```python
from build123d import *

# Parameters (mm, degrees)
SKETCH1_W           = 155
SKETCH1_H           = 55
BOSS_EXTRUDE1_DEPTH = 10
SKETCH2_W           = 143
SKETCH2_H           = 20
CUT_EXTRUDE1_DEPTH  = 5
SKETCH3_W           = 10
SKETCH3_H           = 30
BOSS_EXTRUDE2_DEPTH = 78
SKETCH4_W           = 35
SKETCH4_H           = 20
SKETCH4_W_2         = 50
CUT_EXTRUDE2_DEPTH  = 78
SKETCH5_W           = 155
SKETCH5_H           = 88
BOSS_EXTRUDE3_DEPTH = 15
SKETCH6_W           = 115
SKETCH6_H           = 48
CUT_EXTRUDE3_DEPTH  = 20
SKETCH7_W           = 5
SKETCH7_H           = 58
CUT_EXTRUDE4_DEPTH  = 200
CUT_EXTRUDE5_DEPTH  = 35
SKETCH9_R           = 2
CUT_EXTRUDE6_DEPTH  = 10
SKETCH10_R          = 2
CUT_EXTRUDE7_DEPTH  = 20


with BuildPart() as part:
    # Sketch1 → Boss-Extrude1 (new body)
    with BuildSketch(Plane(origin=(0, 0, 0), x_dir=(1, 0, 0), z_dir=(0, 1, 0))):
        with Locations((77.5, -27.5)):
            Rectangle(SKETCH1_W, SKETCH1_H)
    extrude(amount=BOSS_EXTRUDE1_DEPTH)

    # Sketch2 → Cut-Extrude1 (cut)
    with BuildSketch(Plane(origin=(0, 10, 0), x_dir=(1, 0, 0), z_dir=(0, 1, 0))):
        with Locations((77.5, -15)):
            Rectangle(SKETCH2_W, SKETCH2_H)
    extrude(amount=-CUT_EXTRUDE1_DEPTH, mode=Mode.SUBTRACT)

    # Sketch3 → Boss-Extrude2 (add)
    with BuildSketch(Plane(origin=(0, 10, 0), x_dir=(1, 0, 0), z_dir=(0, 1, 0))):
        with Locations((5, -40)):
            Rectangle(SKETCH3_W, SKETCH3_H)
        with Locations((150, -40)):
            Rectangle(SKETCH3_W, SKETCH3_H)
    extrude(amount=BOSS_EXTRUDE2_DEPTH)

    # Sketch4 → Cut-Extrude2 (cut)
    with BuildSketch(Plane(origin=(0, 5, 0), x_dir=(1, 0, 0), z_dir=(0, 1, 0))):
        with Locations((23.5, -15)):
            Rectangle(SKETCH4_W, SKETCH4_H)
        with Locations((124, -15)):
            Rectangle(SKETCH4_W_2, SKETCH4_H)
    extrude(amount=-CUT_EXTRUDE2_DEPTH, mode=Mode.SUBTRACT)

    # Sketch5 → Boss-Extrude3 (add)
    with BuildSketch(Plane.XY.offset(55)):
        with Locations((77.5, 44)):
            Rectangle(SKETCH5_W, SKETCH5_H)
    extrude(amount=BOSS_EXTRUDE3_DEPTH)

    # Sketch6 → Cut-Extrude3 (cut)
    with BuildSketch(Plane.XY.offset(70)):
        with Locations((77.5, 44)):
            Rectangle(SKETCH6_W, SKETCH6_H)
    extrude(amount=-CUT_EXTRUDE3_DEPTH, mode=Mode.SUBTRACT)

    # Sketch7 → Cut-Extrude4 (cut)
    with BuildSketch(Plane(origin=(155, 0, 0), x_dir=(0, 0, -1), z_dir=(1, 0, 0))):
        with Locations((-62.5, 44)):
            Rectangle(SKETCH7_W, SKETCH7_H)
    extrude(amount=-CUT_EXTRUDE4_DEPTH, mode=Mode.SUBTRACT)

    # Sketch8 → Cut-Extrude5 (cut)
    with BuildSketch(Plane.XY.offset(70)):
        Polygon((47.5, 0), (107.5, 0), (77.5, 50), align=None)
    extrude(amount=-CUT_EXTRUDE5_DEPTH, mode=Mode.SUBTRACT)

    # Sketch9 → Cut-Extrude6 (cut)
    with BuildSketch(Plane(origin=(0, 88, 0), x_dir=(1, 0, 0), z_dir=(0, 1, 0))):
        with Locations((150, -40)):
            Circle(SKETCH9_R)
        with Locations((5, -40)):
            Circle(SKETCH9_R)
    extrude(amount=-CUT_EXTRUDE6_DEPTH, mode=Mode.SUBTRACT)

    # Sketch10 → Cut-Extrude7 (cut)
    with BuildSketch(Plane(origin=(0, 88, 0), x_dir=(1, 0, 0), z_dir=(0, 1, 0))):
        with Locations((109, -62.5)):
            Circle(SKETCH10_R)
        with Locations((46, -62.5)):
            Circle(SKETCH10_R)
    extrude(amount=-CUT_EXTRUDE7_DEPTH, mode=Mode.SUBTRACT)


solid = part.part
```
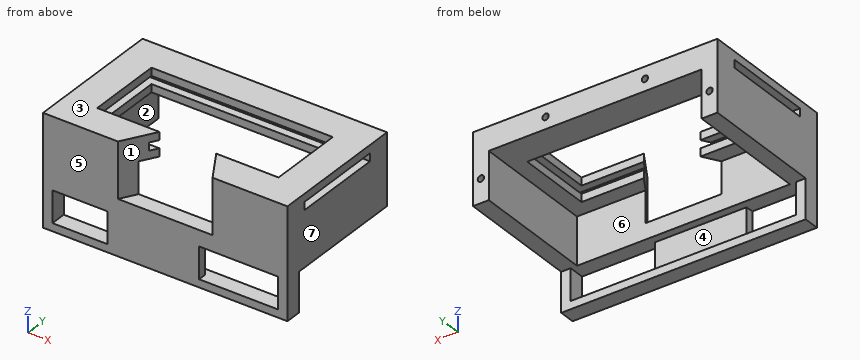
Can you work these out from the model? Positions are in its coordinate system, mm. Face numbers are marked on the shaded views. A direction names the side the tool comes from. Coordinates: 2 decimals unless noted, no trailing zeros. Write each loop counter-clockwise with the first axis right and the second up, starting at its lowest first coordinate (ties: lowest second). Pieces come first, ordered by that corner, then holes. Notation, with made-up numbers: (10.5, 78.25) - (50.5, 78.25) arc R30 ccw to (50.5, 107.25) - close; hole circle Ø11 at (36, 24). An arc over 180 degrees is marked (long way). Return JSON: item names as keys, results as strings.
Q1. I'm going to push flat-ended pins straight in: pin 1 Ø6 at (x, z) = (96.5, 17.5) entering from +Y; pin 2 Ø2 at (x, z) = (5.5, 40) entering from +Y; pin 3 Ø1.5 at (x, z) = (71, 68.5) entering from -Y; pin 4 Ø3 at (x, y) = (96, 65) entering from -Z. Where does each tip first touch, or does it pass through?
Computed values:
{"pin 1": "stops at y = 5", "pin 2": "stops at y = 78", "pin 3": "stops at y = 68", "pin 4": "passes through"}
Q2. If we section it at B-B (y = 59.5): Please give me the cut outline in (x, z), then the cut area to 3 significant figures.
Computed values:
{"outline": "(0, 25) - (10, 25) - (10, 55) - (20, 55) - (20, 60) - (0, 60) - close; (0, 65) - (20, 65) - (20, 70) - (0, 70) - close; (135, 55) - (145, 55) - (145, 25) - (155, 25) - (155, 60) - (135, 60) - close; (135, 65) - (155, 65) - (155, 70) - (135, 70) - close", "area": "1,000 mm2"}
Q3. If we section it at D-D (z = 9): Please give me the cut outline in (x, y).
Computed values:
{"outline": "(0, 0) - (6, 0) - (6, 10) - (0, 10) - close; (41, 0) - (99, 0) - (99, 5) - (41, 5) - close; (149, 0) - (155, 0) - (155, 10) - (149, 10) - close"}
Q4. Thinking about a two-plate mould opening in X: for the marked faces 5, 6 and 7, which applies, +X half, -X half, draft (parallel to the pull), parting line (faces both ways), or undercut?
Computed values:
{"face 5": "draft", "face 6": "undercut", "face 7": "+X half"}
Q5. If we section it at A-A (x = 76.5): Please give me the cut outline in (y, z).
Computed values:
{"outline": "(0, 0) - (10, 0) - (10, 5) - (5, 5) - (5, 25) - (10, 25) - (10, 35) - (0, 35) - close; (68, 55) - (88, 55) - (88, 70) - (68, 70) - (68, 65) - (73, 65) - (73, 60) - (68, 60) - close"}
Q6. If we section it at C-C (z = 40): Please give me the cut outline in (x, y).
Computed values:
{"outline": "(0, 0) - (47.5, 0) - (53.5, 10) - (10, 10) - (10, 88) - (7, 88) - (7, 78) - (3, 78) - (3, 88) - (0, 88) - close; (101.5, 10) - (107.5, 0) - (155, 0) - (155, 88) - (152, 88) - (152, 78) - (148, 78) - (148, 88) - (145, 88) - (145, 10) - close"}
Q7. Please list where these lines run through material, in increasing order: L1, parallel to X at y = 84.75, z = 40; L2, parallel to X at y = 69, z = 37; L3, parallel to Z at x = 109, y = 84.5. Write a range as from..to.
Computed values:
{"L1": "x = 0..3, 7..10, 145..148, 152..155", "L2": "x = 0..10, 145..155", "L3": "z = 55..60.5, 64.5..70"}
Q8. On a 3-axis mill with a long thin cutter (end or side, diameter ignored), from which of +Z, -Z, +X, -X, +Y, -Y can I reach the whole of each face in a straight line? I mean the marked faces 1, 2, 3 and 4. Say none if no direction works.
Computed values:
{"face 1": "+Z, -Y", "face 2": "-Z, +Y", "face 3": "+Z, +X, -X, +Y, -Y", "face 4": "+Y"}
